Input: part model. Units: mm. Frame: model coordinates. Face numbers are marked on the shaded views. Coordinates: 2 decimals unless noted, no trailing zeros. Write each loop counter-clockwise with the first axis right and the second up, starting at its lowest first coordinate (ties: lowest second). Pieces come first, ordered by that corner, then holes.
1) Section query D-D (z = 11). Output: boundary loops of the cut face in (x, y), then the cut area to 3 significant figures.
2) Section query A-A (x = 0). Output: boundary loops of the cut face in (y, z).
3) Line query: L1, parallel to X at y = 1.75, z = 0; L2, parallel to X at y = 46, z = 1.5; L3, parallel to X at y = 16.5, z = -5. Output: solid intervals per line, ascending.
4) Pin query (flat end, axial travel): pin 1 Ø5 at (x, y) = (4, 39) entering from +Z; pin 2 Ø12 at (y, z) = (50, -11.5) entering from -X; pin 3 Ø4 at (y, z) = (56.5, -8) entering from -X. Return the tip coordinate at first contact, or that it passes through.
5) Section query C-C (y = 19.5). Output: boundary loops of the cut face in (x, z), then the cut area to 3 significant figures.
6) Section query B-B (z = 0). Output: boundary loops of the cut face in (x, y), then the cut area to 3 significant figures.
7) Draft query along X for the marked faces 1, 2 and 3. Return one class per face: pulls with the +X half, pulls with the -X half, needs draft (parallel to the pull), parting line crosses it, or undercut.
from build123d import *

# Parameters (mm, degrees)
SKETCH1_R           = 15
SKETCH1_R_2         = 4
BOSS_EXTRUDE1_DEPTH = 67.12
SKETCH1_3_R         = 4
CUT_EXTRUDE1_DEPTH  = 7
SKETCH1_4_R         = 16
SKETCH1_4_R_2       = 15
BOSS_EXTRUDE2_DEPTH = 5


with BuildPart() as part:
    # Sketch1 → Boss-Extrude1 (new body)
    with BuildSketch(Plane(origin=(0, 0, 0), x_dir=(1, 0, 0), z_dir=(0, 1, 0))):
        with Locations(Location((0, 0, 0), (0, 0, 270))):
            Circle(SKETCH1_R)
        Circle(SKETCH1_R_2, mode=Mode.SUBTRACT)
        Circle(SKETCH1_R_2)
    extrude(amount=BOSS_EXTRUDE1_DEPTH)

    # Sketch1_3 → Cut-Extrude1 (cut)
    with BuildSketch(Plane(origin=(0, 0, 0), x_dir=(1, 0, 0), z_dir=(0, 1, 0))):
        with Locations(Location((0, 0, 0), (0, 0, 270))):
            Circle(SKETCH1_3_R)
    extrude(amount=CUT_EXTRUDE1_DEPTH, mode=Mode.SUBTRACT)

    # Sketch1_4 → Boss-Extrude2 (add)
    with BuildSketch(Plane(origin=(0, 0, 0), x_dir=(1, 0, 0), z_dir=(0, 1, 0))):
        with Locations(Location((0, 0, 0), (0, 0, 270))):
            Circle(SKETCH1_4_R)
        with Locations(Location((0, 0, 0), (0, 0, 270))):
            Circle(SKETCH1_4_R_2, mode=Mode.SUBTRACT)
    extrude(amount=BOSS_EXTRUDE2_DEPTH)


solid = part.part
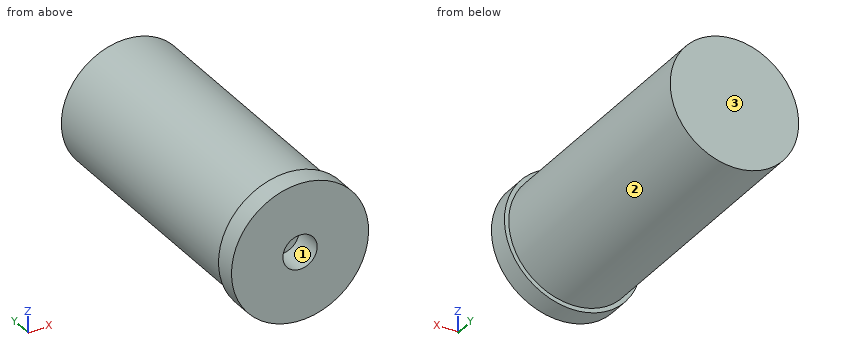
Answer:
1. outline: (-11.62, 0) - (11.62, 0) - (11.62, 5) - (10.2, 5) - (10.2, 67.12) - (-10.2, 67.12) - (-10.2, 5) - (-11.62, 5) - close
1. area: 1,380 mm2
2. outline: (0, -16) - (5, -16) - (5, -15) - (67.12, -15) - (67.12, 15) - (5, 15) - (5, 16) - (0, 16) - (0, 4) - (7, 4) - (7, -4) - (0, -4) - close
3. L1: x = -16 to -4, 4 to 16
3. L2: x = -14.92 to 14.92
3. L3: x = -14.14 to 14.14
4. pin 1: stops at z = 14.92
4. pin 2: stops at x = -13.96
4. pin 3: stops at x = -13.75
5. outline: circle Ø30 at (0, 0)
5. area: 707 mm2
6. outline: (-16, 0) - (-4, 0) - (-4, 7) - (4, 7) - (4, 0) - (16, 0) - (16, 5) - (15, 5) - (15, 67.12) - (-15, 67.12) - (-15, 5) - (-16, 5) - close
6. area: 1,970 mm2
7. face 1: undercut
7. face 2: parting line crosses it
7. face 3: needs draft
